Could you check a few things on this model? Use its own coordinates, in mm. Coordinates: 2 decimals unless noted, no trailing zeros. Order: outer loops, then holes, each group sorted by start corner. A loop starts at its lowest first (then second) coordinate and runs counter-clockwise, first axis right, second up. Notation, with made-up numbers: (-10, 74) -> (7, 74) arc R26 ccw to (7, 99) -> close; hole circle Ø1 at (-33, -17.5). An arc over 180 degrees is marked (long way). Put each result on its own line as item: value. Start each with the question number.
Q1. If we section it at C-C (x = -55): Please give me the cut outline in (y, z), and give its area (3 significant figures).
Q2. If we section it at A-A (x = 47): Please give me the cut outline in (y, z).
Q3. Please list where these lines run through material, in increasing order: line 1 along Y through (x, z) = (47, 1.35); line 2 along X through (y, z) = (-1, 1.55); line 3 along Y through (x, z) = (-38, 0.6).
Q4. If we section it at D-D (z = 0.75): Count the separate pieces of the cut face and the enclosed holes in it, and give its area (3 significant figures).
Q5. Will this pin go through, and if not, where does the flat tip stop? pin 1 (1 mm diameter, centred on y = -44, z = 1.5, fed in from +X).
Q6. If we section it at B-B (y = -2): Please give me the cut outline in (x, z), and give its area (3 significant figures).
from build123d import *

# Parameters (mm, degrees)
SKETCH_1_W          = 176
SKETCH_1_H          = 65
SKETCH_1_R          = 2.1
EXTRUDE_1_DEPTH     = 2
FILLET_1_R          = 3
SKETCH_2_R          = 85
CUT_EXTRUDE_1_DEPTH = 24
SKETCH_4_W          = 50
SKETCH_4_H          = 19.5
EXTRUDE_2_DEPTH     = 2
FILLET_2_R          = 3
SKETCH_3_R          = 1.6
CUT_EXTRUDE_2_DEPTH = 12
FILLET_3_R          = 2
SKETCH_5_R          = 1.6
CUT_EXTRUDE_3_DEPTH = 12
SKETCH_6_R          = 1.6
CUT_EXTRUDE_4_DEPTH = 12
SKETCH_7_W          = 90
SKETCH_7_H          = 32
CUT_EXTRUDE_5_DEPTH = 10
FILLET_4_R          = 10


with BuildPart() as part:
    # 草图1 → 凸台-拉伸1 (new body)
    with BuildSketch(Plane.XY):
        Rectangle(SKETCH_1_W, SKETCH_1_H)
        with Locations((-83, 27)):
            Circle(SKETCH_1_R, mode=Mode.SUBTRACT)
        with Locations((-83, -27)):
            Circle(SKETCH_1_R, mode=Mode.SUBTRACT)
        with Locations(Location((83, -27, 0), (0, 0, 180))):
            Circle(SKETCH_1_R, mode=Mode.SUBTRACT)
        with Locations(Location((83, 27, 0), (0, 0, 180))):
            Circle(SKETCH_1_R, mode=Mode.SUBTRACT)
    extrude(amount=EXTRUDE_1_DEPTH)

    # 圆角1
    fillet_1_edges = [part.edges().sort_by_distance(p)[0] for p in [
        (-88, 32.5, 1),
        (88, 32.5, 1),
        (88, -32.5, 1),
        (-88, -32.5, 1),
    ]]
    fillet(fillet_1_edges, radius=FILLET_1_R)

    # 草图2 → 切除-拉伸1 (cut)
    with BuildSketch(Plane.XY.offset(2)):
        with Locations((0, 107.95)):
            Circle(SKETCH_2_R)
    extrude(amount=-CUT_EXTRUDE_1_DEPTH, mode=Mode.SUBTRACT)

    # 草图4 → 凸台-拉伸2 (add)
    with BuildSketch(Plane.XY.offset(2)):
        with Locations((37, -42.25)):
            Rectangle(SKETCH_4_W, SKETCH_4_H)
    extrude(amount=-EXTRUDE_2_DEPTH)

    # 圆角2
    fillet_2_edges = [part.edges().sort_by_distance(p)[0] for p in [
        (-39.144571782, 32.5, 1),
        (39.144571782, 32.5, 1),
        (12, -52, 1),
        (12, -32.5, 1),
        (62, -32.5, 1),
        (62, -52, 1),
    ]]
    fillet(fillet_2_edges, radius=FILLET_2_R)

    # 草图3 → 切除-拉伸2 (cut)
    with BuildSketch(Plane.XY.offset(2)):
        with Locations((16, 19.5)):
            Circle(SKETCH_3_R)
        with Locations((58, 19.5)):
            Circle(SKETCH_3_R)
        with Locations((58, -43.5)):
            Circle(SKETCH_3_R)
        with Locations((16, -43.5)):
            Circle(SKETCH_3_R)
        Polygon((19, 20.5), (19, 16.5), (15, 16.5), (15, -40.5), (19, -40.5), (19, -44.5), (55, -44.5), (55, -40.5), (59, -40.5), (59, 16.5), (55, 16.5), (55, 20.5), align=None)
    extrude(amount=-CUT_EXTRUDE_2_DEPTH, mode=Mode.SUBTRACT)

    # 圆角3
    fillet_3_edges = [part.edges().sort_by_distance(p)[0] for p in [
        (55, 16.5, 1),
        (59, 16.5, 1),
        (59, -40.5, 1),
        (55, -40.5, 1),
        (55, -44.5, 1),
        (19, -44.5, 1),
        (19, -40.5, 1),
        (15, -40.5, 1),
        (19, 16.5, 1),
        (19, 20.5, 1),
        (55, 20.5, 1),
        (15, 16.5, 1),
    ]]
    fillet(fillet_3_edges, radius=FILLET_3_R - 0.0001)  # a hair under: the kernel refuses the full size

    # 草图5 → 切除-拉伸3 (cut)
    with BuildSketch(Plane.XY.offset(2)):
        with Locations((27, -49)):
            Circle(SKETCH_5_R)
        with Locations((47, -49)):
            Circle(SKETCH_5_R)
    extrude(amount=-CUT_EXTRUDE_3_DEPTH, mode=Mode.SUBTRACT)

    # 草图6 → 切除-拉伸4 (cut)
    with BuildSketch(Plane.XY.offset(2)):
        with Locations((-78, 20.5)):
            Circle(SKETCH_6_R)
        with Locations((-38, 20.5)):
            Circle(SKETCH_6_R)
        with Locations((-38, -19.5)):
            Circle(SKETCH_6_R)
        with Locations((-78, -19.5)):
            Circle(SKETCH_6_R)
    extrude(amount=-CUT_EXTRUDE_4_DEPTH, mode=Mode.SUBTRACT)

    # 草图7 → 切除-拉伸5 (cut)
    with BuildSketch(Plane.XY.offset(2)):
        with Locations((-38, 0.5)):
            Rectangle(SKETCH_7_W, SKETCH_7_H)
    extrude(amount=-CUT_EXTRUDE_5_DEPTH, mode=Mode.SUBTRACT)

    # 圆角4
    fillet_4_edges = [part.edges().sort_by_distance(p)[0] for p in [
        (-83, -15.5, 1),
        (-83, 16.5, 1),
        (7, 16.5, 1),
        (7, -15.5, 1),
    ]]
    fillet(fillet_4_edges, radius=FILLET_4_R)


solid = part.part
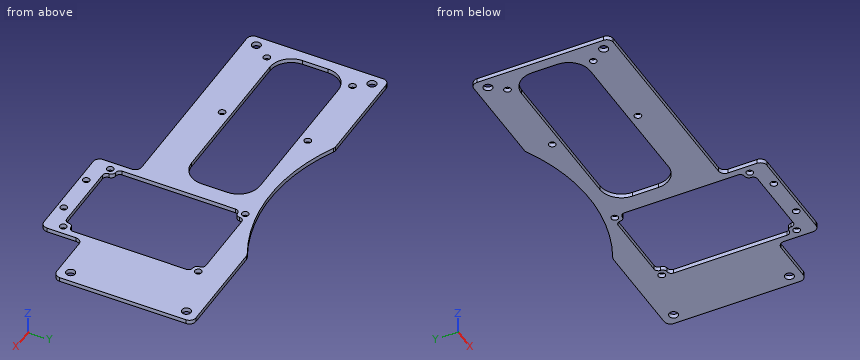
The answers:
1. outline: (-32.5, 0) -> (-15.5, 0) -> (-15.5, 2) -> (-32.5, 2) -> close; (16.5, 0) -> (32.5, 0) -> (32.5, 2) -> (16.5, 2) -> close
1. area: 66.0 mm^2
2. outline: (-52, 0) -> (-50.6, 0) -> (-50.6, 2) -> (-52, 2) -> close; (-47.4, 0) -> (-44.5, 0) -> (-44.5, 2) -> (-47.4, 2) -> close; (20.5, 0) -> (32.5, 0) -> (32.5, 2) -> (20.5, 2) -> close
3. line 1: -52 to -50.6, -47.4 to -44.5, 20.5 to 32.5
3. line 2: -88 to -83, 7 to 15, 59 to 88
3. line 3: -32.5 to -21.1, -17.9 to -15.5, 16.5 to 18.9, 22.1 to 31.92
4. separate pieces: 1
4. enclosed holes: 16
4. area: 6,180 mm^2
5. pin 1: x = 62
6. outline: (-88, 0) -> (-83, 0) -> (-83, 2) -> (-88, 2) -> close; (7, 0) -> (15, 0) -> (15, 2) -> (7, 2) -> close; (59, 0) -> (88, 0) -> (88, 2) -> (59, 2) -> close
6. area: 84.0 mm^2
